Part model, mm, in its own coordinate system. A direction names the side the tool comes from. Round coordinates to 2 decimals unless told otherwise and drop trailing zeros. Write each loop counter-clockwise with the first axis right and the second up, starting at its lowest first coordinate (ties: lowest second). Pieces come first, ordered by that corner, then holes. Notation, with made-up numbers: M 68,6.5 L 106,6.5 A26 cw 106,36.5 Z; hole C 35.25,-34.5 d10. An arc over 180 degrees is marked long. Use a Markdown table: item, result. Add a question column.
1) Which spindle directions (+Z, -Z, +X, -X, +Y, -Y) get a long thin tool onto all of the face, cutting with end or side? Do faces 4 (the face through (-10, 1.205, 0)), 5 (the face through (4.39, -3, 0)), 6 (the face through (7.38, 8.6, 0.2)), 7 (the face through (-6, 7.17, 0)), 8 (the face through (-11.92, -3, 0)). Say none if no direction does.
2) Two-plate mould, pull along Z, no slides. Class faces 1 (the face through (3.89, -3, 0)), 2 (the face through (-4, 2, 3.175)), 3 (the face through (-10.9, 9.4, -1.875)): released by +Z, released by -Z, zero draft, split by the parting line, or undercut.
3) Slice it at A-A on z = -1.25. Write the cut outline in (x, y) (3 decimals).
4) Slice it at C-C on x = 0. Write the cut outline in (y, z) (3 decimals).
5) Slice it at B-B on y = 0. Write the cut outline in (x, z) (3 decimals).
6) Wall check: probe 1 along X at (y, z) = (-4.5, -1.25); probe 2 along Y at (x, z) = (0, -2) (3 decimals); probe 3 along Y at (x, z) = (-6.75, 1.25). Give the ranges that are in metal, low to high.
7) Drop flat-ended pins along their axis: P1, Ø1.5, axis at y = -3.5, z = 0.5, coming from the +X side; P2, Ø1.5, axis at y = -3, z = 0, coming from the -X side; P3, Ø0.6, axis at x = -2, y = -3.5, coming from the -Z side (3 decimals); P4, Ø0.6, axis at x = -2, y = -3.5, coming from the +Z side (3 decimals). Give the stop position or say it passes through.
8) Slice it at D-D on z = 2.75. Write the cut outline in (x, y) (3 decimals), plus the area to 3 significant figures.
```python
from build123d import *

# Parameters (mm, degrees)
SKETCH_1_R                  = 1.205
EXTRUDE_1_DEPTH             = 3.175
SKETCH_2_W                  = 0.5
SKETCH_2_H                  = 3.63
EXTRUDE_2_DEPTH             = 3.08
SKETCH_3_R                  = 0.735
CUT_EXTRUDE_1_DEPTH         = 21.998730652
SKETCH_4_W                  = 6.4
SKETCH_4_H                  = 3.75
CUT_EXTRUDE_2_DEPTH         = 1
SKETCH_6_W                  = 21.4
SKETCH_6_H                  = 3.75
EXTRUDE_3_DEPTH             = 0.5
SKETCH_7_W                  = 3.65
SKETCH_7_H                  = 4.7
EXTRUDE_4_DEPTH             = 0.5
EXTRUDE_5_DEPTH             = 0.5
EXTRUDE_7_REACH             = 22.071
SKETCH_9_R                  = 2.325
EXTRUDE_7_DIRECTION_2_REACH = 22.071


with BuildPart() as part:
    # 스케치1 → 보스-돌출1 (new, symmetric)
    with BuildSketch(Plane.XY):
        Polygon((-14.02, -2.36), (5.82, -2.36), (5.82, 6.58), (-4.42, 6.58), (-5.01, 7.17), (-7.62, 7.17), (-7.62, 9.908), (-14.02, 9.908), (-14.02, 6.58), align=None)
        Circle(SKETCH_1_R, mode=Mode.SUBTRACT)
        with BuildLine():
            Line((-10.212788401, 1.205), (-8.847211599, 1.205))
            ThreePointArc((-8.847211599, 1.205), (-8.145, 0), (-8.847211599, -1.205))
            Line((-8.847211599, -1.205), (-10.212788401, -1.205))
            ThreePointArc((-10.212788401, -1.205), (-10.915, 0), (-10.212788401, 1.205))
        make_face(mode=Mode.SUBTRACT)
    extrude(amount=EXTRUDE_1_DEPTH, both=True)

    # 스케치2 → 보스-돌출2 (add)
    with BuildSketch(Plane.XZ.offset(2.36)):
        with Locations((-12.17, 0)):
            Rectangle(SKETCH_2_W, SKETCH_2_H)
        with Locations((-1.88, 0)):
            Rectangle(SKETCH_2_W, SKETCH_2_H)
        with Locations((4.14, 0)):
            Rectangle(SKETCH_2_W, SKETCH_2_H)
    extrude(amount=EXTRUDE_2_DEPTH)

    # 스케치3 → 컷-돌출1 (cut, through all)
    with BuildSketch(Plane.ZY.offset(12.42)):
        with Locations(Location((0, -3.9, 0), (0, 0, 270))):
            Circle(SKETCH_3_R)
    extrude(amount=-CUT_EXTRUDE_1_DEPTH, mode=Mode.SUBTRACT)

    # 스케치4 → 컷-돌출2 (cut)
    with BuildSketch(Plane(origin=(0, 9.908, 0), x_dir=(1, 0, 0), z_dir=(0, 1, 0))):
        with Locations((-10.82, 0)):
            Rectangle(SKETCH_4_W, SKETCH_4_H)
    extrude(amount=-CUT_EXTRUDE_2_DEPTH, mode=Mode.SUBTRACT)

    # 스케치6 → 보스-돌출3 (add)
    with BuildSketch(Plane(origin=(0, 8.908, 0), x_dir=(1, 0, 0), z_dir=(0, 1, 0))):
        with Locations((-3.32, 0)):
            Rectangle(SKETCH_6_W, SKETCH_6_H)
    extrude(amount=-EXTRUDE_3_DEPTH)

    # 스케치7 → 보스-돌출4 (add)
    with BuildSketch(Plane(origin=(0, 8.908, 0), x_dir=(1, 0, 0), z_dir=(0, 1, 0))):
        with Locations((5.555, 0)):
            Rectangle(SKETCH_7_W, SKETCH_7_H)
    extrude(amount=-EXTRUDE_4_DEPTH)

    # 스케치8 → 보스-돌출5 (add)
    with BuildSketch(Plane.XY.offset(2.35)):
        with BuildLine():
            Line((3.73, 8.408), (7.38, 8.408))
            Line((7.38, 8.408), (7.38, 12.183))
            ThreePointArc((7.38, 12.183), (5.555, 14.008), (3.73, 12.183))
            Line((3.73, 12.183), (3.73, 8.408))
        make_face()
    extrude_5 = extrude(amount=-EXTRUDE_5_DEPTH)

    # 대칭 복사1: 보스-돌출5 across plane
    add(extrude_5.mirror(Plane.XY))

    # 보스-돌출7: up to this face of the body (flat: up to its plane)
    extrude_7_end = Plane(part.part.faces().sort_by_distance((5.555, 11.279795549, 1.85))[0])
    # 스케치9 → 보스-돌출7 (add, up to the picked face)
    with BuildSketch(Plane.XY, mode=Mode.PRIVATE) as extrude_7_sk1:
        with Locations(Location((5.555, 12.183, 0), (0, 0, 218.284293925))):
            Circle(SKETCH_9_R)
    extrude_7_tool1 = split(extrude(extrude_7_sk1.sketch, amount=EXTRUDE_7_REACH, mode=Mode.PRIVATE), bisect_by=extrude_7_end, keep=Keep.BOTH, mode=Mode.PRIVATE)
    add(extrude_7_tool1.solids().sort_by(Axis((5.555, 12.183, 0), (0, 0, 1)))[0])

    # 보스-돌출7 direction 2: up to this face of the body (flat: up to its plane)
    extrude_7_direction_2_end = Plane(part.part.faces().sort_by_distance((5.555, 11.279795549, -1.85))[0])
    # 스케치9 → 보스-돌출7 direction 2 (add, up to the picked face)
    with BuildSketch(Plane.XY, mode=Mode.PRIVATE) as extrude_7_direction_2_sk1:
        with Locations(Location((5.555, 12.183, 0), (0, 0, 218.284293925))):
            Circle(SKETCH_9_R)
    extrude_7_direction_2_tool1 = split(extrude(extrude_7_direction_2_sk1.sketch, amount=-EXTRUDE_7_DIRECTION_2_REACH, mode=Mode.PRIVATE), bisect_by=extrude_7_direction_2_end, keep=Keep.BOTH, mode=Mode.PRIVATE)
    add(extrude_7_direction_2_tool1.solids().sort_by(Axis((5.555, 12.183, 0), (0, 0, -1)))[0])


solid = part.part
```
Entries:
| question | item | result |
|---|---|---|
| 1 | face 4 | +Z, -Z |
| 1 | face 5 | +Z, -Z, +X, -Y |
| 1 | face 6 | +X, -Y |
| 1 | face 7 | +Z, -Z, +X |
| 1 | face 8 | +Z, -Z, -Y |
| 2 | face 1 | zero draft |
| 2 | face 2 | released by +Z |
| 2 | face 3 | undercut |
| 3 | outline | M -14.02,-2.36 L -12.42,-2.36 L -12.42,-5.44 L -11.92,-5.44 L -11.92,-2.36 L -2.13,-2.36 L -2.13,-5.44 L -1.63,-5.44 L -1.63,-2.36 L 3.89,-2.36 L 3.89,-5.44 L 4.39,-5.44 L 4.39,-2.36 L 5.82,-2.36 L 5.82,6.58 L -4.42,6.58 L -5.01,7.17 L -7.62,7.17 L -7.62,8.408 L 7.38,8.408 L 7.38,8.908 L -14.02,8.908 Z; C 5.555,12.183 d4.65; hole M -10.213,-1.205 L -8.847,-1.205 A1.385 ccw -8.847,1.205 L -10.213,1.205 A1.385 ccw Z; hole C 0,0 d2.41 |
| 4 | outline | M -2.36,-3.175 L -1.205,-3.175 L -1.205,3.175 L -2.36,3.175 Z; M 1.205,-3.175 L 6.58,-3.175 L 6.58,3.175 L 1.205,3.175 Z; M 8.408,-1.875 L 8.908,-1.875 L 8.908,1.875 L 8.408,1.875 Z |
| 5 | outline | M -14.02,-3.175 L -10.915,-3.175 L -10.915,3.175 L -14.02,3.175 Z; M -8.145,-3.175 L -1.205,-3.175 L -1.205,3.175 L -8.145,3.175 Z; M 1.205,-3.175 L 5.82,-3.175 L 5.82,3.175 L 1.205,3.175 Z |
| 6 | probe 1 | x = -12.42 to -11.92, -2.13 to -1.63, 3.89 to 4.39 |
| 6 | probe 2 | y = -2.36 to -1.205, 1.205 to 6.58 |
| 6 | probe 3 | y = -2.36 to 7.17, 8.41 to 8.91 |
| 7 | P1 | stops at x = 4.39 |
| 7 | P2 | stops at x = -14.02 |
| 7 | P3 | stops at z = -1.815 |
| 7 | P4 | stops at z = 1.815 |
| 8 | outline | M -14.02,-2.36 L 5.82,-2.36 L 5.82,6.58 L -4.42,6.58 L -5.01,7.17 L -7.62,7.17 L -7.62,9.908 L -14.02,9.908 Z; hole M -10.213,-1.205 L -8.847,-1.205 A1.385 ccw -8.847,1.205 L -10.213,1.205 A1.385 ccw Z; hole C 0,0 d2.41 |
| 8 | area | 190 mm^2 |
